For this review, take the finished solid that the model builds, in its own axes (mm). Face numbers are marked on the shaded views. Give positions to 0.01 mm unless a question says otherwise; leave off trailing zeros. Loops run counter-clockwise (first coordinate to the right, second up) from the corner with the lowest first, then second, coordinate; pieces in that order, holes last. Notation, with made-up numbers: (64, -13) - (79, -13) arc R27 ccw to (79, 3) - close; hole circle Ø2 at (51, 23). An arc over 180 degrees is marked (long way). Put each result on its own line as item: value.
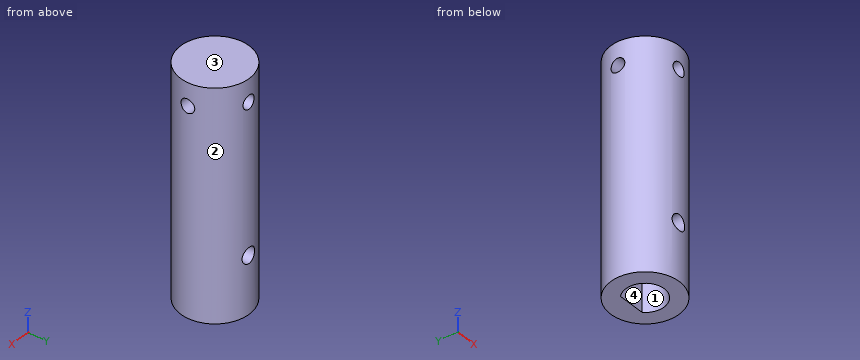
Autodesk Inventor part; units mm, degrees
ref_plane "作業平面1" through (7.5, 0, 0) normal (1, 0, 0) x (0, 1, 0)
ref_plane "作業平面2" through (-7.5, 0, 0) normal (1, 0, 0) x (0, 1, 0)
ref_plane "作業平面3" through (0, 7.5, 0) normal (0, 1, 0) x (-1, 0, 0)
sketch "スケッチ1" plane through (0, 0, 0) normal (0, 0, 1) x (1, 0, 0)
  circle A0 centre (0, 0) radius 7.5
  dimension "d0" = 15
extrude "押し出し1" add sketch "スケッチ1" along normal blind 50
sketch "スケッチ2" plane through (0, 0, 0) normal (0, 0, -1) x (-1, 0, 0)
  arc A0 (-2.9394, 3) -> (2.9394, 3) centre (0, 0) ccw
  line L0 (-2.9394, 3) -> (2.9394, 3)
  point P0 (-3.1305, 2.8)
  dimension "d3" = 4.2
  dimension "d4" = 3
extrude "押し出し2" cut sketch "スケッチ2" against normal blind 30
ref_plane "作業平面1" through (7.5, 0, 0) normal (1, 0, 0) x (0, 1, 0)
ref_plane "作業平面2" through (-7.5, 0, 0) normal (1, 0, 0) x (0, 1, 0)
ref_plane "作業平面3" through (0, 7.5, 0) normal (0, 1, 0) x (-1, 0, 0)
ref_plane "作業平面4" through (0, -7.5, 0) normal (0, 1, 0) x (-1, 0, 0)
sketch "スケッチ3" plane through (7.5, 0, 0) normal (1, 0, 0) x (0, 1, 0)
  circle A0 centre (0, 45) radius 1.5
  line L0 (7.5, 50) -> (-7.5, 50)
  point P0 (0, 0)
  dimension "d11" = 3
  dimension "d12" = 5
sketch "スケッチ4" plane through (-7.5, 0, 0) normal (1, 0, 0) x (0, 1, 0)
  circle A0 centre (0, 45) radius 1.5
  line L0 (7.5, 50) -> (-7.5, 50)
  point P0 (0, 0)
  dimension "d13" = 3
  dimension "d14" = 5
extrude "押し出し3" cut sketch "スケッチ3" against normal blind 5
extrude "押し出し4" cut sketch "スケッチ4" along normal blind 5
sketch "スケッチ5" plane through (0, 7.5, 0) normal (0, 1, 0) x (-1, 0, 0)
  circle A0 centre (0, 45) radius 1.5
  line L0 (7.5, 50) -> (-7.5, 50)
  point P0 (0, 0)
  dimension "d19" = 3
  dimension "d20" = 5
sketch "スケッチ6" plane through (0, -7.5, 0) normal (0, 1, 0) x (-1, 0, 0)
  circle A0 centre (0, 45) radius 1.5
  line L0 (7.5, 50) -> (-7.5, 50)
  point P0 (0, 0)
  dimension "d21" = 3
  dimension "d22" = 5
extrude "押し出し5" cut sketch "スケッチ5" against normal blind 5
extrude "押し出し6" cut sketch "スケッチ6" along normal blind 5
thread "ねじ1"
thread "ねじ2"
thread "ねじ3"
thread "ねじ4"
sketch "スケッチ7" plane through (0, 7.5, 0) normal (0, 1, 0) x (-1, 0, 0)
  circle A0 centre (0, 12.5) radius 1.7
  point P0 (0, 0)
  dimension "d35" = 3.4
  dimension "d36" = 12.5
extrude "押し出し7" cut sketch "スケッチ7" against normal through all
properties part number "rotary_transfer_shaft_5" material "ステンレス鋼"
1) Wall thickness on line 1 (Z direction, x = 0, y = -4.9); line 2 (Z direction, x = -4.8, y = 0); line 3 (X direction, y = 0.25, z = 4.5): over which ranges is each line inside the solid? List them lowest first.
Geometry check:
line 1: z = 0 to 10.8, 14.2 to 43.5, 46.5 to 50
line 2: z = 0 to 43.5, 46.5 to 50
line 3: x = -7.5 to -4.19, 4.19 to 7.5
2) Take a section at A-A on x = 0. State the section outline as (y, z) points, and give its area (3 significant figures).
Geometry check:
outline: (-7.5, 0) - (-4.2, 0) - (-4.2, 10.8) - (-7.5, 10.8) - close; (-7.5, 14.2) - (-4.2, 14.2) - (-4.2, 30) - (3, 30) - (3, 14.2) - (7.5, 14.2) - (7.5, 43.5) - (2.5, 43.5) - (2.5, 46.5) - (7.5, 46.5) - (7.5, 50) - (-7.5, 50) - (-7.5, 46.5) - (-2.5, 46.5) - (-2.5, 43.5) - (-7.5, 43.5) - close; (3, 0) - (7.5, 0) - (7.5, 10.8) - (3, 10.8) - close
area: 477 mm²
3) Take a section at B-B on y = 0. State the section outline as (x, z) points, and give its area (3 significant figures).
Geometry check:
outline: (-7.5, 0) - (-4.2, 0) - (-4.2, 30) - (4.2, 30) - (4.2, 0) - (7.5, 0) - (7.5, 43.5) - (2.5, 43.5) - (2.5, 46.5) - (7.5, 46.5) - (7.5, 50) - (-7.5, 50) - (-7.5, 46.5) - (-2.5, 46.5) - (-2.5, 43.5) - (-7.5, 43.5) - close
area: 468 mm²
4) Draft analysis for pull direction X (two halves, no side actions). For the marked faces 1, 2, 3 and 4, state which applies: pulls with the +X half, pulls with the -X half, needs draft (parallel to the pull), parting line crosses it, or undercut.
Geometry check:
face 1: undercut
face 2: parting line crosses it
face 3: needs draft
face 4: undercut
5) Insertion check: pin 1 Ø3 at (y, z) = (-2.5, 12.5) entering from -X; pin 2 Ø2 at (x, y) = (0.5, -1.5) entering from -Z; pin 3 Ø3.5 at (y, z) = (0, 45) entering from -X; pin 4 Ø2.5 at (y, z) = (0, 45) entering from +X. Each pin has a flat end and moves straight along its axis. Give the tip position at first contact, or say it passes through.
Geometry check:
pin 1: stops at x = -7.43
pin 2: stops at z = 30
pin 3: stops at x = -7.5
pin 4: stops at x = 2.5
6) Take a section at C-C on z = 12.5. State the section outline as (x, y) points, and give its area (3 significant figures).
Geometry check:
outline: (-2.94, 3) - (-1.7, 3) - (-1.7, 7.3) arc R7.5 ccw to (-1.7, -7.3) - (-1.7, -3.84) arc R4.2 cw to start; (1.7, -7.3) arc R7.5 ccw to (1.7, 7.3) - (1.7, 3) - (2.94, 3) arc R4.2 cw to (1.7, -3.84) - close
area: 99.7 mm²
7) Take a section at D-D on z = 6. State the section outline as (x, y) points.
Geometry check:
outline: circle Ø15 at (0, 0); hole (-2.94, 3) arc R4.2 ccw (long way) to (2.94, 3) - close
